The listing builds one solid part. Answer for the finished solid, in the listing's coordinates (mm). A direction names the side the tool comes from. Coordinates: 2 decimals unless noted, no trailing zeros. Loops run counter-clockwise (first coordinate to the right, second up) from the corner with the lowest first, then second, coordinate; pieces in that order, holes last. Notation, with made-up numbers: (76, 53) - (111, 53) arc R33 ccw to (111, 85) - close; hole circle Ø6 at (-40, 24). An arc over 180 degrees is marked (long way). Put each result on its own line as item: value.
```python
from build123d import *

# Parameters (mm, degrees)
SKETCH1_R           = 3.937
BOSS_EXTRUDE1_DEPTH = 3.175


with BuildPart() as part:
    # Sketch1 → Boss-Extrude1 (new body)
    with BuildSketch(Plane.XY):
        with BuildLine():
            Line((93.755372783, 56.217862378), (-93.755372783, 56.217862378))
            ThreePointArc((-93.755372783, 56.217862378), (-98.330168366, 54.924590712), (-101.550779975, 51.427596704))
            ThreePointArc((-101.550779975, 51.427596704), (-113.823339918, 1.267243548), (-102.670596612, -49.153913451))
            ThreePointArc((-102.670596612, -49.153913451), (-90.230339267, -63.122833424), (-72.258999564, -68.311443769))
            Line((-72.258999564, -68.311443769), (72.258999564, -68.311443769))
            ThreePointArc((72.258999564, -68.311443769), (90.230339267, -63.122833424), (102.670596612, -49.153913451))
            ThreePointArc((102.670596612, -49.153913451), (113.823339918, 1.267243548), (101.550779975, 51.427596704))
            ThreePointArc((101.550779975, 51.427596704), (98.330168366, 54.924590712), (93.755372783, 56.217862378))
        make_face()
        with Locations((0, -22.231680406)):
            Circle(SKETCH1_R, mode=Mode.SUBTRACT)
        with Locations((-19.2532, 11.115840203)):
            Circle(SKETCH1_R, mode=Mode.SUBTRACT)
        with Locations((19.2532, 11.115840203)):
            Circle(SKETCH1_R, mode=Mode.SUBTRACT)
        with BuildLine():
            Line((50.537610963, -51.271802519), (24.921430241, -51.271802519))
            ThreePointArc((24.921430241, -51.271802519), (10.088644213, -39.88245969), (17.262248757, -22.612020516))
            ThreePointArc((17.262248757, -22.612020516), (27.847341492, -5.815004372), (24.868702617, 13.81435247))
            ThreePointArc((24.868702617, 13.81435247), (22.438574631, 26.570482702), (30.438512771, 36.799137076))
            ThreePointArc((30.438512771, 36.799137076), (45.320271887, 42.430959459), (61.111403686, 44.386549975))
            ThreePointArc((61.111403686, 44.386549975), (70.335617903, 41.69195489), (76.601720977, 34.406152063))
            ThreePointArc((76.601720977, 34.406152063), (81.115925355, 23.793617751), (82.657376867, 12.364363491))
            ThreePointArc((82.657376867, 12.364363491), (82.169800307, 10.456907156), (80.826687149, 9.017404598))
            ThreePointArc((80.826687149, 9.017404598), (79.903262527, 8.142769936), (79.366676242, 6.98961167))
            ThreePointArc((79.366676242, 6.98961167), (79.918421039, 4.432989113), (82.285769804, 3.321053391))
            ThreePointArc((82.285769804, 3.321053391), (83.453127799, 2.865261142), (83.956280763, 1.717520598))
            ThreePointArc((83.956280763, 1.717520598), (82.285769804, -16.752881668), (76.601720977, -34.406152063))
            ThreePointArc((76.601720977, -34.406152063), (66.06007852, -46.687651069), (50.537610963, -51.271802519))
        make_face(mode=Mode.SUBTRACT)
        with BuildLine():
            Line((-50.537610963, -51.271802519), (-24.921430241, -51.271802519))
            ThreePointArc((-24.921430241, -51.271802519), (-10.088644213, -39.88245969), (-17.262248757, -22.612020516))
            ThreePointArc((-17.262248757, -22.612020516), (-27.847341492, -5.815004372), (-24.868702617, 13.81435247))
            ThreePointArc((-24.868702617, 13.81435247), (-22.438574631, 26.570482702), (-30.438512771, 36.799137076))
            ThreePointArc((-30.438512771, 36.799137076), (-45.320271887, 42.430959459), (-61.111403686, 44.386549975))
            ThreePointArc((-61.111403686, 44.386549975), (-70.335617903, 41.69195489), (-76.601720977, 34.406152063))
            ThreePointArc((-76.601720977, 34.406152063), (-81.115925355, 23.793617751), (-82.657376867, 12.364363491))
            ThreePointArc((-82.657376867, 12.364363491), (-82.169800307, 10.456907156), (-80.826687149, 9.017404598))
            ThreePointArc((-80.826687149, 9.017404598), (-79.903262527, 8.142769936), (-79.366676242, 6.98961167))
            ThreePointArc((-79.366676242, 6.98961167), (-79.918421039, 4.432989113), (-82.285769804, 3.321053391))
            ThreePointArc((-82.285769804, 3.321053391), (-83.453127799, 2.865261142), (-83.956280763, 1.717520598))
            ThreePointArc((-83.956280763, 1.717520598), (-82.285769804, -16.752881668), (-76.601720977, -34.406152063))
            ThreePointArc((-76.601720977, -34.406152063), (-66.06007852, -46.687651069), (-50.537610963, -51.271802519))
        make_face(mode=Mode.SUBTRACT)
    extrude(amount=BOSS_EXTRUDE1_DEPTH)


solid = part.part
```
1) Each of these flat-tipped pins is pushed along its axis until it touches: pin 1 (9 mm diameter, centred on x = -19.25, y = 11.12, fed in from -Z); pin 2 (7 mm diameter, centred on x = 19.25, y = 11.12, fed in from +Z). Where does it stop, or does it pass through?
Found:
pin 1: stops at z = 0
pin 2: passes through
2) The part is cut by section C-C (x = -39.5). Give the vertices of the cut face in (y, z) (3 decimals), and give its area (3 significant figures).
Found:
outline: (-68.311, 0) - (-51.272, 0) - (-51.272, 3.175) - (-68.311, 3.175) - close; (40.707, 0) - (56.218, 0) - (56.218, 3.175) - (40.707, 3.175) - close
area: 103 mm^2
3) The part is cut by section A-A (x = 0). Give the vertices of the cut face in (y, z) (3 decimals), and give its area (3 significant figures).
Found:
outline: (-68.311, 0) - (-26.169, 0) - (-26.169, 3.175) - (-68.311, 3.175) - close; (-18.295, 0) - (56.218, 0) - (56.218, 3.175) - (-18.295, 3.175) - close
area: 370 mm^2
4) The part is cut by section B-B (y = 29). Give the vertices of the cut face in (x, z) (3 decimals), and give its area (3 significant figures).
Found:
outline: (-110.074, 0) - (-79.321, 0) - (-79.321, 3.175) - (-110.074, 3.175) - close; (-23.242, 0) - (23.242, 0) - (23.242, 3.175) - (-23.242, 3.175) - close; (79.321, 0) - (110.074, 0) - (110.074, 3.175) - (79.321, 3.175) - close
area: 343 mm^2
5) The part is cut by section D-D (y = -39). Give the vertices of the cut face in (x, z) (3 decimals).
Found:
outline: (-106.941, 0) - (-74.004, 0) - (-74.004, 3.175) - (-106.941, 3.175) - close; (-9.881, 0) - (9.881, 0) - (9.881, 3.175) - (-9.881, 3.175) - close; (74.004, 0) - (106.941, 0) - (106.941, 3.175) - (74.004, 3.175) - close
6) For faces 4 (the face through (81.073, 23.95, 1.565)), 5 (the face through (-2, -5, 3.175)), determine the directions among +Z, -Z, +X, -X, +Y, -Y from which every point of the face is accessible in a straight line to the end or side of a thin tool.
Found:
face 4: +Z, -Z
face 5: +Z, +X, -X, +Y, -Y
7) For a pull along Y with two mould halves and no side action, classify faces 1 (the face through (66.252, -46.562, 1.565)), 2 (the face through (-90.454, -62.981, 1.565)), 3 (the face through (-2, -5, 0)) as pulls with the +Y half, pulls with the -Y half, needs draft (parallel to the pull), parting line crosses it, or undercut.
Found:
face 1: undercut
face 2: pulls with the -Y half
face 3: needs draft
8) Straight lines are drawn through the part: L1, parallel to Y at x = 0, z = 1.8; L2, parallel to Y at x = 24, z = 2.8; L3, parallel to X at y = -39, z = 2.45. For each, find the intervals that lie inside material, in ascending order. Write a range as [from, to].
Found:
L1: y = [-68.31, -26.17], [-18.29, 56.22]
L2: y = [-68.31, -51.24], [-15.27, 15.19], [30.55, 56.22]
L3: x = [-106.94, -74], [-9.88, 9.88], [74, 106.94]
